The model under review builds one solid part; all positions refer to its coordinate system, in mm. A direction names the side the tool comes from. Give positions to 0.01 mm unless a question says otherwise; leave off trailing zeros. Order: outer loops, then holes, each group sorted by start corner. A loop starts at its lowest first (then second) coordinate and runs counter-clockwise, first axis right, second up. Notation, with made-up numbers: (-0.75, -10) - (44.25, -10) arc R37 ccw to (44.25, 28) - close; hole circle Ø6 at (-33.5, 77.5). An arc over 180 degrees is marked (long way). Use a Markdown table: item, result. Add a question column.
```python
from build123d import *

# Parameters (mm, degrees)
SKETCH2_W               = 50.8
SKETCH2_H               = 75.9206
SKETCH2_W_2             = 44.8564
SKETCH2_H_2             = 69.977
CUT_EXTRUDE1_DEPTH      = 25.4
CUT_EXTRUDE2_DEPTH      = 25.4
BOSS_EXTRUDE1_REACH     = 967.2
SKETCH7_W               = 50.8
SKETCH7_H               = 75.9206
CUT_EXTRUDE3_DEPTH      = 25.4
SKETCH11_W              = 44.8564
SKETCH11_H              = 69.977
CUT_EXTRUDE4_DEPTH      = 482.6
CUT_EXTRUDE4_DEPTH_BACK = 482.6
BOSS_EXTRUDE2_DEPTH     = 75.9206
SKETCH13_W              = 44.8564
SKETCH13_H              = 69.977
CUT_EXTRUDE5_DEPTH      = 279.4
CUT_EXTRUDE5_DEPTH_BACK = 279.4
CUT_EXTRUDE6_DEPTH      = 25.4
FILLET2_R               = 4.191
FILLET3_R               = 4.191


with BuildPart() as part:
    # Sweep1: sweep along a path in Sketch3
    with BuildLine(Plane(origin=(0, 0, 0), x_dir=(1, 0, 0), z_dir=(0, 1, 0))) as sweep1_path:
        Line((0, -204.200684232), (0, 1395.206939042))
        Line((0, 1395.206939042), (382.5875, 1624.599315768))
        Line((382.5875, 1624.599315768), (633.4125, 1624.599315768))
        Line((633.4125, 1624.599315768), (1016, 1395.206939042))
        Line((1016, 1395.206939042), (1016, -204.200684232))
        Line((1016, -204.200684232), (0, -204.200684232))
    # Sketch2 → Sweep1 (sweep)
    with BuildSketch(Plane.XY):
        with Locations((25.4, 37.9603)):
            Rectangle(SKETCH2_W, SKETCH2_H)
        with Locations((25.4, 37.9603)):
            Rectangle(SKETCH2_W_2, SKETCH2_H_2, mode=Mode.SUBTRACT)
    sweep(path=sweep1_path.line, transition=Transition.RIGHT)

    # Sketch4 → Cut-Extrude1 (cut)
    with BuildSketch(Plane.XZ):
        with BuildLine():
            Line((469.9508, 188.312984232), (546.0492, 188.312984232))
            ThreePointArc((546.0492, 188.312984232), (555.5615, 178.800684232), (546.0492, 169.288384232))
            Line((546.0492, 169.288384232), (469.9508, 169.288384232))
            ThreePointArc((469.9508, 169.288384232), (460.4385, 178.800684232), (469.9508, 188.312984232))
        make_face()
    extrude(amount=-CUT_EXTRUDE1_DEPTH, mode=Mode.SUBTRACT)

    # Sketch5 → Cut-Extrude2 (cut)
    with BuildSketch(Plane.XZ):
        with BuildLine():
            Line((469.9, -1589.687015768), (546.1, -1589.687015768))
            ThreePointArc((546.1, -1589.687015768), (555.6123, -1599.199315768), (546.1, -1608.711615768))
            Line((546.1, -1608.711615768), (469.9, -1608.711615768))
            ThreePointArc((469.9, -1608.711615768), (460.3877, -1599.199315768), (469.9, -1589.687015768))
        make_face()
    extrude(amount=-CUT_EXTRUDE2_DEPTH, mode=Mode.SUBTRACT)

    # Sketch7 → Boss-Extrude1 (add, up to next)
    with BuildSketch(Plane.ZY.offset(-965.2), mode=Mode.PRIVATE) as boss_extrude1_sk1:
        with Locations((-202.199315768, 37.9603)):
            Rectangle(SKETCH7_W, SKETCH7_H)
    boss_extrude1_tool1 = extrude(boss_extrude1_sk1.sketch, amount=BOSS_EXTRUDE1_REACH, mode=Mode.PRIVATE) - part.part
    add(boss_extrude1_tool1.solids().sort_by_distance((965.2, 37.9603, -202.199316))[0])

    # Sketch8 → Cut-Extrude3 (cut)
    with BuildSketch(Plane.XZ):
        with BuildLine():
            Line((469.9508, -192.687015768), (546.0492, -192.687015768))
            ThreePointArc((546.0492, -192.687015768), (555.5615, -202.199315768), (546.0492, -211.711615768))
            Line((546.0492, -211.711615768), (469.9508, -211.711615768))
            ThreePointArc((469.9508, -211.711615768), (460.4385, -202.199315768), (469.9508, -192.687015768))
        make_face()
    extrude(amount=-CUT_EXTRUDE3_DEPTH, mode=Mode.SUBTRACT)

    # Sketch11 → Cut-Extrude4 (cut, two sides)
    with BuildSketch(Plane(origin=(508, 0, 0), x_dir=(0, 0, -1), z_dir=(1, 0, 0))) as cut_extrude4_sk:
        with Locations((202.199315768, 37.9603)):
            Rectangle(SKETCH11_W, SKETCH11_H)
    extrude(amount=CUT_EXTRUDE4_DEPTH, mode=Mode.SUBTRACT)
    extrude(cut_extrude4_sk.sketch, amount=-CUT_EXTRUDE4_DEPTH_BACK, mode=Mode.SUBTRACT)

    # Sketch12 → Boss-Extrude2 (add)
    with BuildSketch(Plane(origin=(0, 0, 0), x_dir=(1, 0, 0), z_dir=(0, 1, 0))):
        Polygon((320.396677865, 1528.079315768), (695.603322135, 1528.079315768), (780.329088864, 1477.279315768), (235.670911136, 1477.279315768), align=None)
    extrude(amount=BOSS_EXTRUDE2_DEPTH)

    # Sketch13 → Cut-Extrude5 (cut, two sides)
    with BuildSketch(Plane(origin=(508, 0, 0), x_dir=(0, 0, -1), z_dir=(1, 0, 0))) as cut_extrude5_sk:
        with Locations((1502.679315768, 37.9603)):
            Rectangle(SKETCH13_W, SKETCH13_H)
    extrude(amount=CUT_EXTRUDE5_DEPTH, mode=Mode.SUBTRACT)
    extrude(cut_extrude5_sk.sketch, amount=-CUT_EXTRUDE5_DEPTH_BACK, mode=Mode.SUBTRACT)

    # Sketch14 → Cut-Extrude6 (cut)
    with BuildSketch(Plane.XZ):
        with BuildLine():
            Line((469.9508, -1493.167015768), (546.0492, -1493.167015768))
            ThreePointArc((546.0492, -1493.167015768), (555.5615, -1502.679315768), (546.0492, -1512.191615768))
            Line((546.0492, -1512.191615768), (469.9508, -1512.191615768))
            ThreePointArc((469.9508, -1512.191615768), (460.4385, -1502.679315768), (469.9508, -1493.167015768))
        make_face()
    extrude(amount=-CUT_EXTRUDE6_DEPTH, mode=Mode.SUBTRACT)

    # Fillet2
    fillet2_edges = [part.edges().sort_by_distance(p)[0] for p in [
        (1016, 37.9603, -1395.206939042),
        (0, 37.9603, -1395.206939042),
        (633.4125, 37.9603, -1624.599315768),
        (382.5875, 37.9603, -1624.599315768),
    ]]
    fillet(fillet2_edges, radius=FILLET2_R)

    # Fillet3
    fillet3_edges = [part.edges().sort_by_distance(p)[0] for p in [
        (235.670911136, 37.9603, -1477.279315768),
        (780.329088864, 37.9603, -1477.279315768),
        (50.8, 37.9603, -1366.434142591),
        (968.1718, 37.9603, -1368.117351183),
    ]]
    fillet(fillet3_edges, radius=FILLET3_R)


solid = part.part
```
Q1. We need section A-A (z = -1094). Write out the cut boundary in (x, y).
Q2. Wall thickness on probe 1 along X at (y, z) = (9.5, -274.5); probe 2 along Z at (x, y) = (784, 40); probe 3 along Z at (x, y) = (232.5, 70.5): over which ranges is each line inside the solid? List them lowest first.
Q3. We need section B-B (y = 30.5). Count the separate pieces of the cut face and the enclosed holes in it, plus the area to 3 significant figures.
Q4. Clearance check with flat-ended pins moving along their axes: P1, Ø1.5, axis at x = 686.5, y = 32.5, coming from the -Z side; P2, Ø10, axis at x = 910, y = 27.5, coming from the -Z side. State where each tip first meets the part, or that it passes through.
Q5. Machinability: for faces 1 (the flat face through (502, 37, 153.401)), 2 (the flat face through (874.939, 38.45, -1424.018)), 3 (the flat face through (194.471, 38.492, -1511.808)), which of the approach directions +Z, -Z, +X, -X, +Y, -Y give a long, thin tool a straight path to every point of the face, cutting with its end or side? Answer none if there is none.
Q6. We need section C-C (x = 204.5). Write out the cut boundary in (y, z).
Q7. Draft analysis for pull direction Z (two halves, no side actions). For faces 4 (the flat face through (510, 38, -1624.599)), 5 (the flat face through (1000, 75.921, -647)), 6 (the flat face through (502, 38, 156.372)), state which applies: pulls with the +Z half, pulls with the -Z half, needs draft (parallel to the pull), parting line crosses it, or undercut.
Here are the results:
| question | item | result |
|---|---|---|
| 1 | outline | (0, 0) - (50.8, 0) - (50.8, 75.92) - (0, 75.92) - close; (965.2, 0) - (1016, 0) - (1016, 75.92) - (965.2, 75.92) - close; hole (2.97, 2.97) - (47.83, 2.97) - (47.83, 72.95) - (2.97, 72.95) - close; hole (968.17, 2.97) - (1013.03, 2.97) - (1013.03, 72.95) - (968.17, 72.95) - close |
| 2 | probe 1 | 0 to 2.97, 47.83 to 50.8, 965.2 to 968.17, 1013.03 to 1016 |
| 2 | probe 2 | -1534.31 to -1530.84, -1478.54 to -1475.08, -227.6 to -224.63, -179.77 to -176.8, 153.4 to 156.37, 201.23 to 204.2 |
| 2 | probe 3 | -1534.61 to -1531.14, -1478.84 to -1475.38, -227.6 to -224.63, -179.77 to -176.8, 153.4 to 156.37, 201.23 to 204.2 |
| 3 | separate pieces | 4 |
| 3 | enclosed holes | 4 |
| 3 | area | 38,100 mm2 |
| 4 | P1 | z = -1593.22 |
| 4 | P2 | z = -1461.76 |
| 5 | face 1 | +Y, -Y |
| 5 | face 2 | none |
| 5 | face 3 | -Z, -X, +Y, -Y |
| 6 | outline | (0, -1517.82) - (75.92, -1517.82) - (75.92, -1458.59) - (0, -1458.59) - close; (0, -227.6) - (75.92, -227.6) - (75.92, -176.8) - (0, -176.8) - close; (0, 153.4) - (75.92, 153.4) - (75.92, 204.2) - (0, 204.2) - close; hole (2.97, -1514.36) - (72.95, -1514.36) - (72.95, -1462.05) - (2.97, -1462.05) - close; hole (2.97, -224.63) - (72.95, -224.63) - (72.95, -179.77) - (2.97, -179.77) - close; hole (2.97, 156.37) - (72.95, 156.37) - (72.95, 201.23) - (2.97, 201.23) - close |
| 7 | face 4 | pulls with the -Z half |
| 7 | face 5 | needs draft |
| 7 | face 6 | undercut |
